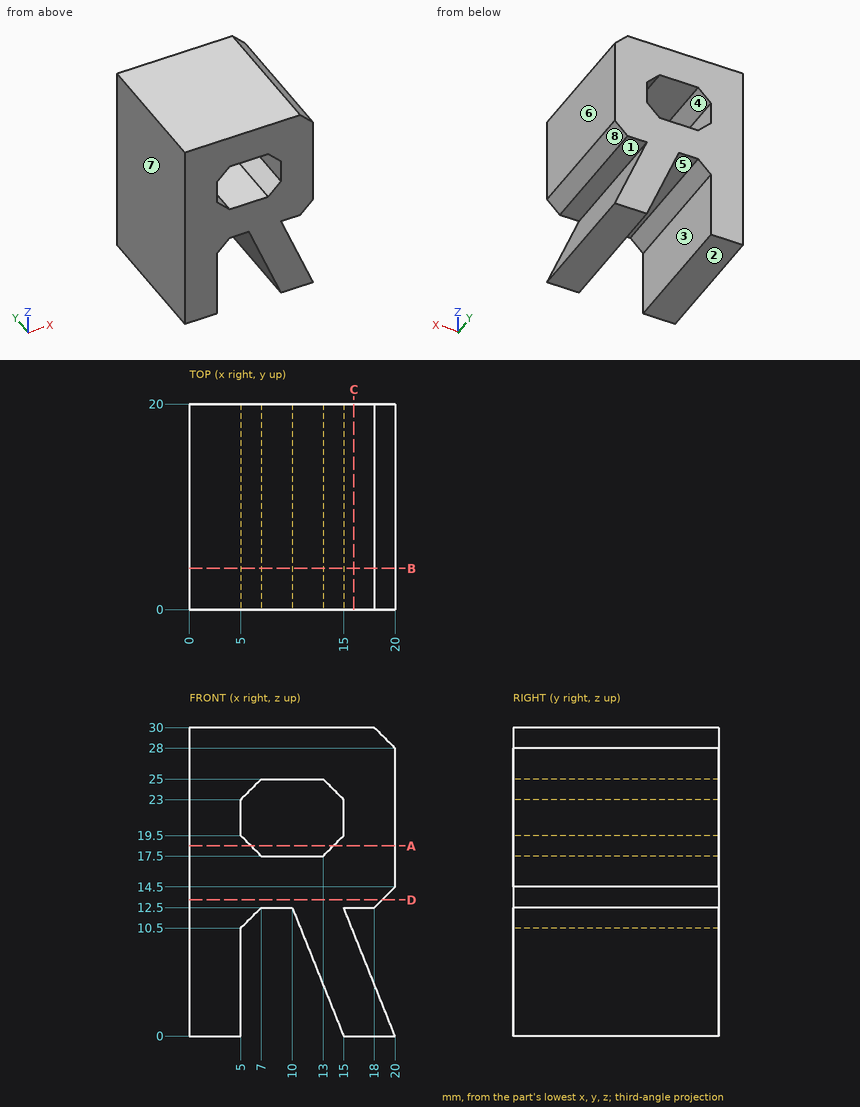
Can you work these out from the drawing? Everything is in mm from the part's minimum corner. A direction names the side the tool comes from. Give positions to 0.01 mm unless a question says otherwise; leave off trailing zeros. Order: outer loops, then holes, each group sorted by start corner. A loop starts at its lowest first (then second) coordinate and runs counter-clockwise, first axis right, second up. Notation, with made-up numbers: (20, 1.5) -> (54, 1.5) arc R9 cw to (54, 13.5) -> close; hole circle Ø5 at (-28.75, 14). An arc over 180 degrees is marked (long way). Return JSON: item names as keys, results as strings.
1. Thinking about a two-plate mould opening in Z: for the marked faces 1, 2 and 3, which applies, pulls with the +Z half, pulls with the -Z half, needs draft (parallel to the pull), parting line crosses it, or undercut?
Answer list:
{"face 1": "undercut", "face 2": "pulls with the -Z half", "face 3": "needs draft"}
2. I need wall thicknesses on line 1 (X direction, y = 3, z = 23); line 2 (Z direction, x = 7.5, y = 14.5); line 3 (X direction, y = 2.5, z = 7.5). Which ranges of each line are inside material? Lowest first, please. Write a range as from..to.
Answer list:
{"line 1": "x = 0..5, 15..20", "line 2": "z = 12.5..17.5, 25..30", "line 3": "x = 0..5, 12..17"}
3. On a 3-axis mill with a long thin cutter (end or side, diameter ignored), from which of +Z, -Z, +X, -X, +Y, -Y can I reach the whole of each face in a straight line? I mean the marked faces 4, 5, 6, 7 and 8. Say none if no direction works.
Answer list:
{"face 4": "+Y, -Y", "face 5": "-Z, +Y, -Y", "face 6": "+Z, -Z, +X, +Y, -Y", "face 7": "+Z, -Z, -X, +Y, -Y", "face 8": "+X, +Y, -Y"}
4. Imagine slicing it at C-C on x = 16. List the corners of the cut face in (y, z) for me.
Answer list:
{"outline": "(0, 0) -> (20, 0) -> (20, 10) -> (0, 10) -> close; (0, 12.5) -> (20, 12.5) -> (20, 30) -> (0, 30) -> close"}
5. Imagine slicing it at D-D on z = 13.25. List the corners of the cut face in (x, y) for me.
Answer list:
{"outline": "(0, 0) -> (18.75, 0) -> (18.75, 20) -> (0, 20) -> close"}
6. For pin 1 Ø3 at (y, z) = (6.5, 3.5) entering from +X; pin 2 Ø5 at (x, y) = (9, 5.5) entering from -Z; pin 3 Ø2 at (y, z) = (5, 4) entering from +X, each with a flat end and sliding along its axis, tell me the tip position at first contact or that it passes through.
Answer list:
{"pin 1": "stops at x = 19.2", "pin 2": "stops at z = 8.75", "pin 3": "stops at x = 18.8"}
7. Imagine slicing it at B-B on y = 4. List the corners of the cut face in (x, z) for me, then the cut area to 3 significant figures.
Answer list:
{"outline": "(0, 0) -> (5, 0) -> (5, 10.5) -> (7, 12.5) -> (10, 12.5) -> (15, 0) -> (20, 0) -> (15, 12.5) -> (18, 12.5) -> (20, 14.5) -> (20, 28) -> (18, 30) -> (0, 30) -> close; hole (5, 19.5) -> (7, 17.5) -> (13, 17.5) -> (15, 19.5) -> (15, 23) -> (13, 25) -> (7, 25) -> (5, 23) -> close", "area": "406 mm2"}
8. Imagine slicing it at A-A on z = 18.5. List the corners of the cut face in (x, y) for me.
Answer list:
{"outline": "(0, 0) -> (6, 0) -> (6, 20) -> (0, 20) -> close; (14, 0) -> (20, 0) -> (20, 20) -> (14, 20) -> close"}
